```python
from build123d import *

# Parameters (mm, degrees)
F0_W     = 63.5
F0_H     = 44.45
F1_DEPTH = 38.1
F2_W     = 31.75
F2_H     = 13.187168
F3_DEPTH = 9.525
F4_W     = 63.5
F4_H     = 19.05
F5_DEPTH = 19.05
F6_W     = 25.4
F6_H     = 12.7
F7_DEPTH = 63.501


with BuildPart() as f1:
    # F0 (on Front) → F1 (new body)
    with BuildSketch(Plane.XZ):
        Rectangle(F0_W, F0_H)
    extrude(amount=F1_DEPTH)

    # F2 (on face) → F3 (cut)
    with BuildSketch(Plane.XZ.offset(38.1)):
        with Locations((0, 15.631416)):
            Rectangle(F2_W, F2_H)
    extrude(amount=-F3_DEPTH, mode=Mode.SUBTRACT)

    # F4 (on face) → F5 (cut)
    with BuildSketch(Plane.XY.offset(22.225)):
        with Locations((0, -19.05)):
            Rectangle(F4_W, F4_H)
    extrude(amount=-F5_DEPTH, mode=Mode.SUBTRACT)

    # F6 (on face) → F7 (cut, through all)
    with BuildSketch(Plane.YZ.offset(31.75)):
        with Locations((-19.05, -15.875)):
            Rectangle(F6_W, F6_H)
    extrude(amount=-F7_DEPTH, mode=Mode.SUBTRACT)


solid = f1.part
```
Verification items for the finished model (mm, model axes). A direction names the side the tool comes from. Round coordinates to 2 decimals unless told otherwise and drop trailing zeros. Write each loop counter-clockwise with the first axis right and the second up, starting at its lowest first coordinate (ties: lowest second). Pieces come first, ordered by that corner, then holes.
1. Section check A-A on z = -18.5. Enter the section's corners in (x, y).
2. Scan lines: L1, parallel to Y at x = 29.5, z = 16 (3 decimals); L2, parallel to Y at x = -23, z = -18; L3, parallel to Z at x = 22.5, y = -12 (3 decimals). Record each from-to range of solid material in increasing order.
3. Access from +Z, -Z, +X, -X, +Y, -Y to the whole of each face (thin tool, end or side, straight path). Record for faces 4 (the flat face through (0, -31.75, -16)), 5 (the flat face through (15.875, -33, 16)), 6 (the flat face through (0, -9.525, 13)), 7 (the flat face through (31.75, -19, 0)), 8 (the flat face through (0, -5, 22.225)).
4. Section check D-D on y = -21.5. Enter the section's corners in (x, z) (3 decimals).
5. Draft check along X on faces 1 (the flat face through (-31.75, -19, 0)), 2 (the flat face through (0, -33, 9.038)), 3 (the flat face through (0, -19, -9.525)). Enter one of: +X half, -X half, draft (parallel to the pull), parting line (faces both ways), or undercut.
6. Gauge pin test, flat ends, axial feed: P1, Ø3, axis at x = 2.5, y = -35, coming from the +Z side; P2, Ø2, axis at x = 16, y = -27.5, coming from the -Z side (3 decimals). Record the tip position at first contact, or that the pin passes through.
7. Section check B-B on x = 13.5. Enter the section's corners in (y, z) (3 decimals).
8. Section check C-C on z = 15. Enter the section's corners in (x, y) (3 decimals).
Answer:
1. outline: (-31.75, -38.1) - (31.75, -38.1) - (31.75, -31.75) - (-31.75, -31.75) - close; (-31.75, -6.35) - (31.75, -6.35) - (31.75, 0) - (-31.75, 0) - close
2. L1: y = -38.1 to -28.575, -9.525 to 0
2. L2: y = -38.1 to -31.75, -6.35 to 0
2. L3: z = -9.525 to 3.175
3. face 4: -Z, +X, -X
3. face 5: +Z, -Y
3. face 6: +Z, +X, -X
3. face 7: +Z, -Z, +X, +Y, -Y
3. face 8: +Z, +X, -X, +Y, -Y
4. outline: (-31.75, -9.525) - (31.75, -9.525) - (31.75, 3.175) - (-31.75, 3.175) - close
5. face 1: -X half
5. face 2: undercut
5. face 3: draft
6. P1: stops at z = 9.04
6. P2: stops at z = -9.525
7. outline: (-38.1, -22.225) - (-31.75, -22.225) - (-31.75, -9.525) - (-6.35, -9.525) - (-6.35, -22.225) - (0, -22.225) - (0, 22.225) - (-9.525, 22.225) - (-9.525, 3.175) - (-28.575, 3.175) - (-28.575, 9.038) - (-38.1, 9.038) - close
8. outline: (-31.75, -38.1) - (-15.875, -38.1) - (-15.875, -28.575) - (-31.75, -28.575) - close; (-31.75, -9.525) - (31.75, -9.525) - (31.75, 0) - (-31.75, 0) - close; (15.875, -38.1) - (31.75, -38.1) - (31.75, -28.575) - (15.875, -28.575) - close
